Could you check a few things on this model? Use its own coordinates, in mm. Coordinates: 2 decimals unless noted, no trailing zeros. Order: outer loops, then holes, each group sorted by start corner. A loop starts at its lowest first (then second) coordinate and runs counter-clockwise, first axis right, second up. Notation, with made-up numbers: (5.5, 72) - (39.5, 72) arc R7 cw to (39.5, 76) - close; hole circle Ø5 at (74, -34.75). An arc over 180 degrees is marked (long way). Answer as CSV lines item,"result". Start each with the question number.
1. I want a section at A-A, the plane x = 0. List the corners of the cut face in (y, z) for me, and give its area (3 significant figures).
2. I need wall thicknesses on probe 1 along X at (y, z) = (-21.5, 1.45) (3 decimals); probe 2 along Y at (x, z) = (-4.5, 3.05); probe 3 along Y at (x, z) = (-8.5, 2.7). Which ranges of each line are inside material? Lowest first, please.
3. For pin 1 (1.5 mm diameter, centred on x = -5, z = 1.5, fed in from -Y); pin 2 (1.5 mm diameter, centred on x = 5, z = 1.5, fed in from +Y); pin 3 (4 mm diameter, centred on x = -5, y = 21, fed in from -Z), each with a flat end and sliding along its axis, tell me the tip position at first contact or that it passes through.
4. I want a section at B-B, the plane x = 8.7. List the corners of the cut face in (y, z) for me, and give its area (3 significant figures).
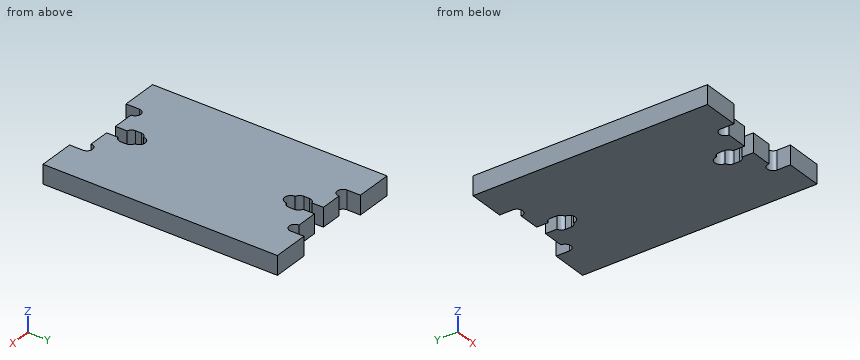
Solid Edge part; units mm, degrees
sketch "Sketch1" plane through (0, 0, 0) normal (0, 0, 1) x (1, 0, 0)
  line L0 (-10.2, 27.5) -> (10.2, 27.5)
  line L1 (10.2, 27.5) -> (10.2, 31)
  line L2 (19.8, 31) -> (10.2, 31)
  line L3 (19.8, 31) -> (19.8, -31)
  line L4 (10.2, -31) -> (19.8, -31)
  line L5 (10.2, -27.5) -> (10.2, -31)
  line L6 (-10.2, -27.5) -> (10.2, -27.5)
  line L7 (-10.2, -27.5) -> (-10.2, -31)
  line L8 (-10.2, -31) -> (-19.8, -31)
  line L9 (-19.8, 31) -> (-19.8, -31)
  line L10 (-10.2, 31) -> (-19.8, 31)
  line L11 (-10.2, 27.5) -> (-10.2, 31)
extrude "Protrusion1" add sketch "Sketch1" along normal blind 5
sketch "Sketch2" plane through (0, 0, 5) normal (0, 0, 1) x (1, 0, 0)
  circle A0 centre (8.7, 27.5) radius 1.5
  circle A1 centre (-8.7, 27.5) radius 1.5
  circle A2 centre (8.7, -27.5) radius 1.5
  circle A3 centre (-8.7, -27.5) radius 1.5
extrude "ExtrudedCutout_4" cut sketch "Sketch2" against normal blind 5
sketch "Sketch3" plane through (0, 0, 0) normal (0, 0, -1) x (0, 1, 0)
  line L0 (-27.5, -1.5998) -> (-24.4524, -1.5998)
  arc A0 (-24.4524, -1.5998) -> (-23, -2.725) centre (-23, -1.225) ccw
  line L1 (-23, -2.725) -> (-21.5, -2.725)
  arc A1 (-21.5, -2.725) -> (-20.0476, -1.5998) centre (-21.5, -1.225) ccw
  arc A2 (-20.0476, 1.5998) -> (-20.0476, -1.5998) centre (-20.0254, 0) cw
  arc A3 (-21.5, 2.725) -> (-20.0476, 1.5998) centre (-21.5, 1.225) cw
  line L2 (-23, 2.725) -> (-21.5, 2.725)
  arc A4 (-24.4524, 1.6) -> (-23, 2.725) centre (-23, 1.225) cw
  line L3 (-27.5, 1.6) -> (-24.4524, 1.6)
  line L4 (-27.5, 0) -> (-27.5, 1.6)
  line L5 (-27.5, 0) -> (-27.5, -1.5998)
  arc A5 (21.5, 2.725) -> (20.0476, 1.5998) centre (21.5, 1.225) ccw
  arc A6 (20.0476, 1.5998) -> (20.0476, -1.5998) centre (20.0254, 0) ccw
  arc A7 (21.5, -2.725) -> (20.0476, -1.5998) centre (21.5, -1.225) cw
  line L6 (23, -2.725) -> (21.5, -2.725)
  arc A8 (24.4524, -1.5998) -> (23, -2.725) centre (23, -1.225) cw
  line L7 (27.5, -1.5998) -> (24.4524, -1.5998)
  line L8 (27.5, 0) -> (27.5, -1.5998)
  line L9 (27.5, 0) -> (27.5, 1.6)
  line L10 (27.5, 1.6) -> (24.4524, 1.6)
  arc A9 (24.4524, 1.6) -> (23, 2.725) centre (23, 1.225) ccw
  line L11 (23, 2.725) -> (21.5, 2.725)
extrude "Cutout1" cut sketch "Sketch3" against normal up to next
properties material "Polycarbonate"
Solved:
1,outline,"(-18.43, 0) - (18.43, 0) - (18.43, 5) - (-18.43, 5) - close"
1,area,"184 mm2"
2,probe 1,"x = -19.8 to -2.725, 2.725 to 19.8"
2,probe 2,"y = -27.5 to 27.5"
2,probe 3,"y = -26.01 to 26.01"
3,pin 1,"stops at y = -27.5"
3,pin 2,"stops at y = 27.5"
3,pin 3,"stops at z = 0"
4,outline,"(-26, 0) - (26, 0) - (26, 5) - (-26, 5) - close"
4,area,"260 mm2"
